The figure shows three views and two pictorial views of one solid part (mm, origin at its lowest corner). Answer the questions. A direction names the side the tool comes from. Round coordinates to 2 decimals unless told otherwise and drop trailing zeros. Order: outer loops, then holes, each group sorted by start corner. A loop starts at its lowest first (then second) coordinate and runs counter-clockwise, first axis right, second up. Notation, with made-up numbers: (45, 10) - (80, 10) arc R19 ccw to (80, 22) - close; hole circle Ø4 at (67, -3). An arc over 180 degrees is marked (long way). Answer in a Markdown table with one row per item.
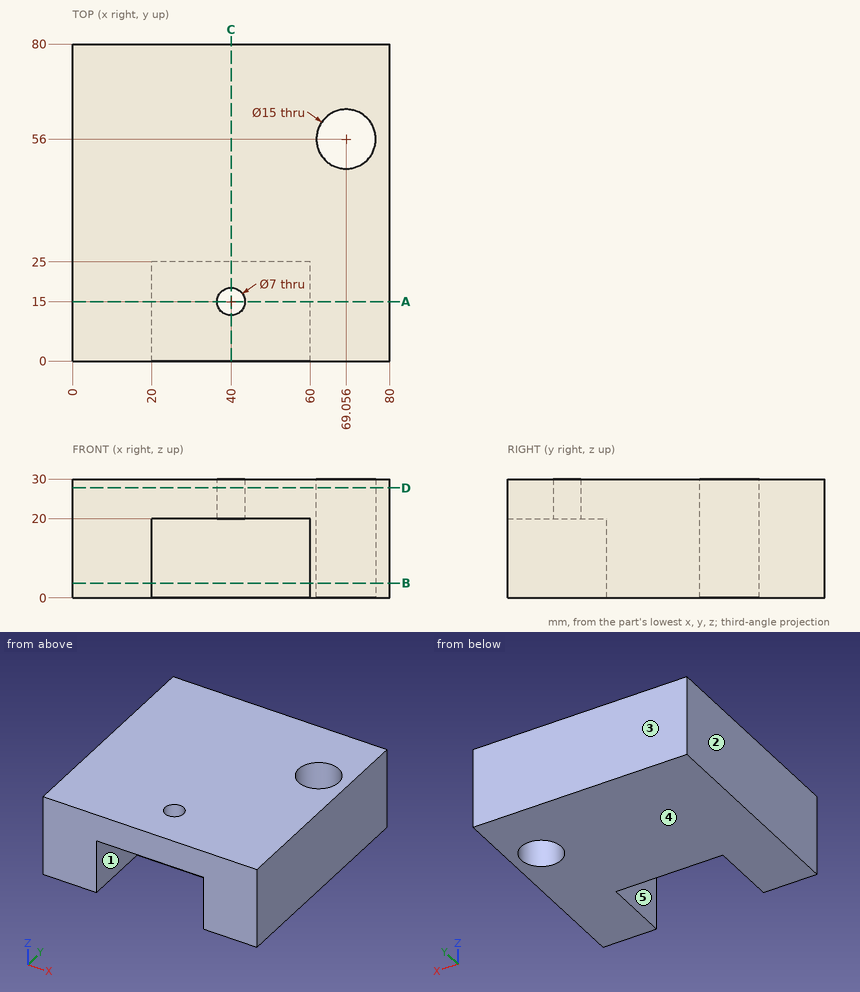
1) Find section C-C, the plane x = 40. Give the vertices of the cut face in (y, z).
Filled in:
| item | result |
|---|---|
| outline | (0, 20) - (11.5, 20) - (11.5, 30) - (0, 30) - close; (18.5, 20) - (25, 20) - (25, 0) - (80, 0) - (80, 30) - (18.5, 30) - close |
2) Which of the six approach directions +Z, -Z, +X, -X, +Y, -Y give full straight-line access (tool end or side, diameter ignored) to the marked faces 4 and 5?
Filled in:
| item | result |
|---|---|
| face 4 | -Z, +X, -X, +Y, -Y |
| face 5 | -Z, -Y |
3) Find section B-B, the plane z = 3.75. Give the vertices of the cut face in (x, y), then the cut area to 3 significant figures.
Filled in:
| item | result |
|---|---|
| outline | (0, 0) - (20, 0) - (20, 25) - (60, 25) - (60, 0) - (80, 0) - (80, 80) - (0, 80) - close; hole circle Ø15 at (69.06, 56) |
| area | 5,220 mm^2 |
4) The mould has two halves that part along X. Classify the marked faces 1, 2 and 3: released by +X, released by -X, zero draft, split by the parting line, or undercut.
Filled in:
| item | result |
|---|---|
| face 1 | undercut |
| face 2 | released by -X |
| face 3 | zero draft |
5) Find section A-A, the plane y = 15. Give the vertices of the cut face in (x, z), then the cut area to 3 significant figures.
Filled in:
| item | result |
|---|---|
| outline | (0, 0) - (20, 0) - (20, 20) - (36.5, 20) - (36.5, 30) - (0, 30) - close; (43.5, 20) - (60, 20) - (60, 0) - (80, 0) - (80, 30) - (43.5, 30) - close |
| area | 1,530 mm^2 |
6) Find the intervals of material crossed by probe 1 along X at (y, z) = (13.5, 12); probe 2 along Y at (x, z) = (40, 25); probe 3 along Y at (x, z) = (25, 16.75), in increasing order. Write a range as from..to.
Filled in:
| item | result |
|---|---|
| probe 1 | x = 0..20, 60..80 |
| probe 2 | y = 0..11.5, 18.5..80 |
| probe 3 | y = 25..80 |
7) Find section D-D, the plane z = 27.75. Give the vertices of the cut face in (x, y).
Filled in:
| item | result |
|---|---|
| outline | (0, 0) - (80, 0) - (80, 80) - (0, 80) - close; hole circle Ø7 at (40, 15); hole circle Ø15 at (69.06, 56) |
8) This flat-tipped pin is pushed along its axis until it touches: pin 1 (12.5 mm diameter, centred on x = 47, y = 8, fed in from -Z). Where does it stop, or does it pass through?
Filled in:
| item | result |
|---|---|
| pin 1 | stops at z = 20 |
